Part model, mm, in its own coordinate system. A direction names the side the tool comes from. Give positions to 0.01 mm unless a question says otherwise; leave off trailing zeros. Order: outer loops, then holes, each group sorted by start corner. A loop starts at its lowest first (then second) coordinate and runs counter-clockwise, first axis right, second up. Notation, with made-up numbers: M 56.25,81.25 L 75.25,81.25 A6 cw 75.25,85.25 Z; hole C -3.75,9.5 d10. An arc over 180 degrees is marked long. Return JSON: item names as keys, results as strings.
from build123d import *

# Parameters (mm, degrees)
CHAMFER1_SIZE  = 1
CHAMFER1_SIZE2 = 0.577350269


with BuildPart() as part:
    # Sketch1 → Revolve1 (revolve)
    with BuildSketch(Plane.XY, mode=Mode.PRIVATE) as revolve1_sk:
        Polygon((16, 2), (9, 2), (8.75, 2), (8.75, 17), (6.75, 17), (6.75, 6.533333333), (2.5, 2), (0, 2), (0, 0), (16, 0), align=None)
        Polygon((6.75, 2), (6.75, 5.466666667), (3.5, 2), align=None, mode=Mode.SUBTRACT)
    revolve(revolve1_sk.sketch.rotate(Axis((0, 21.623043933, 0), (0, -1, 0)), 90), axis=Axis((0, 21.623043933, 0), (0, -1, 0)))

    # Chamfer1
    chamfer1_edges = [part.edges().sort_by_distance(p)[0] for p in [
        (0, 17, -8.75),
    ]]
    chamfer1_side = [part.faces().sort_by_distance(p)[0] for p in [
        (0, 9.5, -8.75),
    ]]
    chamfer(chamfer1_edges, length=CHAMFER1_SIZE, length2=CHAMFER1_SIZE2, reference=chamfer1_side[0])


solid = part.part
Q1. Band-saw the part on D-D (y = 1). Give the cut face in (x, z), then the cut area to 3 significant figures.
Established:
{"outline": "C 0,0 d32", "area": "804 mm²"}
Q2. Pin check, flat tips, straight feed: pin 1 (5 mm diameter, centred on x = 0.5, y = 15, fed in from -Z); pin 2 (1 mm diameter, centred on x = -9, z = 10.5, fed in from +Y); pin 3 (8 mm diameter, centred on x = 3.5, z = -0.5, fed in from -Y); pin 4 (4 mm diameter, centred on x = -1, z = 0, fed in from +Y). Stop position of each tip, or through.
Established:
{"pin 1": "stops at z = -8.75", "pin 2": "stops at y = 2", "pin 3": "stops at y = 0", "pin 4": "stops at y = 2.53"}
Q3. Band-saw the part on A-A (x = 0). Give the cut face in (y, z).
Established:
{"outline": "M 0,-16 L 2,-16 L 2,-8.75 L 16,-8.75 L 17,-8.17 L 17,-6.75 L 6.53,-6.75 L 2,-2.5 L 2,2.5 L 6.53,6.75 L 17,6.75 L 17,8.17 L 16,8.75 L 2,8.75 L 2,16 L 0,16 Z; hole M 2,-6.75 L 5.47,-6.75 L 2,-3.5 Z; hole M 2,3.5 L 5.47,6.75 L 2,6.75 Z"}
Q4. Two-plate mould, pull along Y, no slides. Class faces 4 (the cylindrical face through (6.59, 11.69, -1.46)), 5 (the conical face through (2.64, 2.22, -0.59)), 6 (the flat face through (3, 2, -3)): +Y half, -Y half, draft (parallel to the pull), parting line (faces both ways), or undercut.
Established:
{"face 4": "draft", "face 5": "+Y half", "face 6": "undercut"}
Q5. Band-saw the part on C-C (y = 12.75). Give the cut face in (x, z), then the cut area to 3 significant figures.
Established:
{"outline": "C 0,0 d17.5; hole C 0,0 d13.5", "area": "97.4 mm²"}
Q6. Probe line 1 along X through (y, z) = (10.75, 0); line 2 along X through (y, z) = (3.6, 0); line 3 along X through (y, z) = (3.25, -1). List the from-to ranges inside material, lowest first.
Established:
{"line 1": "x = -8.75 to -6.75, 6.75 to 8.75", "line 2": "x = -8.75 to -6.75, -5 to -4, 4 to 5, 6.75 to 8.75", "line 3": "x = -8.69 to -6.68, -4.56 to -3.53, 3.53 to 4.56, 6.68 to 8.69"}
Q7. 3-axis set-ups, long thin cutter, end or side, ignore diameter. For faces 1 (the cylindrical face through (6.59, 3.76, -1.46)), 2 (the flat face through (7, 2, 7)), 3 (the cylindrical face through (15.62, 1.01, -3.47)): which of +Z, -Z, +X, -X, +Y, -Y reach the whole face in a straight line?
Established:
{"face 1": "none", "face 2": "+Y", "face 3": "+Y, -Y"}
Q8. Band-saw the part on B-B (z = 0). Give the cut face in (x, y), then the cut area to 3 significant figures.
Established:
{"outline": "M -16,0 L 16,0 L 16,2 L 8.75,2 L 8.75,16 L 8.17,17 L 6.75,17 L 6.75,6.53 L 2.5,2 L -2.5,2 L -6.75,6.53 L -6.75,17 L -8.17,17 L -8.75,16 L -8.75,2 L -16,2 Z; hole M -6.75,2 L -3.5,2 L -6.75,5.47 Z; hole M 3.5,2 L 6.75,2 L 6.75,5.47 Z", "area": "131 mm²"}
